Input: part model. Units: mm. Frame: model coordinates. A direction names the side the tool comes from. Give positions to 0.01 mm unless a question says otherwise; leave off trailing zeros. Loops run counter-clockwise (first coordinate to the right, second up) from the corner with the lowest first, then second, coordinate; pieces in that order, holes last.
Solid Edge part; units mm, degrees
sketch "Sketch1" plane through (0, 0, 25) normal (0, 0, 1) x (1, 0, 0)
  line L0 (-49.5, -36.5) -> (-19.5, -36.5)
  line L1 (-19.5, 6.5) -> (-19.5, -36.5)
  line L2 (-19.5, 6.5) -> (-49.5, 6.5)
  line L3 (-49.5, 6.5) -> (-49.5, -36.5)
  circle A0 centre (-25, -31) radius 2.2
  circle A1 centre (-44, 1) radius 2.2
  circle A2 centre (-25, 1) radius 2.2
  circle A3 centre (-44, -31) radius 2.2
extrude "ExtrudedProtrusion_1" add sketch "Sketch1" along normal blind 15
sketch "Sketch2" plane through (-34.5, -36.5, 32.5) normal (0, -1, 0) x (0, 0, 1)
  circle A0 centre (-7.5, 0) radius 4
extrude "Cutout1" cut sketch "Sketch2" against normal through all
sketch "Sketch3" plane through (-34.5, -36.5, 32.5) normal (0, -1, 0) x (1, 0, 0)
  line L0 (-5, 7.5) -> (-5, 4.5)
  line L1 (-5, 4.5) -> (5, 4.5)
  line L2 (5, 7.5) -> (5, 4.5)
  dimension "D1" = 5
  dimension "D2" = 5
extrude "Cutout2" cut sketch "Sketch3" against normal through all material side at (-39.45, -36.5, 38.5)
sketch "Sketch4" plane through (-24.5, -15, 40) normal (0, 0, 1) x (0, 1, 0)
  line L0 (-10.5, 25) -> (-10.5, 12.5)
extrude "Cutout3" cut sketch "Sketch4" against normal through all material side at (-43.25, -25.45, 40)
fillet "Round_1" radius 1 2 edges at (-39.5, -31, 37) (-29.5, -31, 37)
sketch "Sketch5" plane through (-44.5, -31, 40) normal (0, 0, 1) x (1, 0, 0)
  line L0 (0.5, 0) -> (2.0825, 1.5282)
  line L1 (2.0825, 1.5282) -> (0.5, 3.167)
  line L2 (0.5, 3.167) -> (-1.0825, 1.5282)
  line L3 (-1.0825, 1.5282) -> (0.5, 0)
  line L4 (19.5, 0) -> (21.0825, 1.5282)
  line L5 (21.0825, 1.5282) -> (19.5, 3.167)
  line L6 (19.5, 3.167) -> (17.9175, 1.5282)
  line L7 (17.9175, 1.5282) -> (19.5, 0)
extrude "Cutout4" cut sketch "Sketch5" against normal through all
properties material "ABS Plastic, medium impact"
(1) Cut plane A-A (z = 32). Return the cut outline in (x, y), and give its area (3 significant figures).
Values follow:
outline: (-49.5, -36.5) - (-19.5, -36.5) - (-19.5, -25.5) - (-49.5, -25.5) - close; hole (-45.57, -29.46) arc R2.2 ccw (long way) to (-42.43, -29.46) - (-44, -27.83) - close; hole (-26.57, -29.46) arc R2.2 ccw (long way) to (-23.43, -29.46) - (-25, -27.83) - close
area: 297 mm2
(2) Pin query (flat end, axial travel): pin 1 Ø2 at (x, y) = (-32.5, -29) entering from -Z; pin 2 Ø1.5 at (x, y) = (-35, -35) entering from +Z. Return the tip coordinate at first contact, or that it passes through.
Values follow:
pin 1: stops at z = 27.65
pin 2: stops at z = 37
(3) Cut plane B-B (y = -31). Return the cut outline in (x, z), and give its area (3 significant figures).
Values follow:
outline: (-49.5, 25) - (-46.2, 25) - (-46.2, 40) - (-49.5, 40) - close; (-41.8, 25) - (-38.5, 25) arc R4 cw to (-30.5, 25) - (-27.2, 25) - (-27.2, 40) - (-29.5, 40) - (-29.5, 38) arc R1 cw to (-30.5, 37) - (-38.5, 37) arc R1 cw to (-39.5, 38) - (-39.5, 40) - (-41.8, 40) - close; (-22.8, 25) - (-19.5, 25) - (-19.5, 40) - (-22.8, 40) - close
area: 263 mm2
(4) Ray query, probe 1 along X at (y, z) = (-31, 31.5); probe 2 along X at (y, z) = (-29.75, 26); probe 3 along X at (y, z) = (-31, 37.75). Return the intervals inside material, ascending.
Values follow:
probe 1: x = -49.5 to -46.2, -41.8 to -27.2, -22.8 to -19.5
probe 2: x = -49.5 to -45.81, -42.19 to -38.37, -30.63 to -26.81, -23.19 to -19.5
probe 3: x = -49.5 to -46.2, -41.8 to -39.47, -29.53 to -27.2, -22.8 to -19.5
(5) Cut plane C-C (z = 27.5). Return the cut outline in (x, y).
Values follow:
outline: (-49.5, -36.5) - (-37.62, -36.5) - (-37.62, -25.5) - (-49.5, -25.5) - close; (-31.38, -36.5) - (-19.5, -36.5) - (-19.5, -25.5) - (-31.38, -25.5) - close; hole (-45.57, -29.46) arc R2.2 ccw (long way) to (-42.43, -29.46) - (-44, -27.83) - close; hole (-26.57, -29.46) arc R2.2 ccw (long way) to (-23.43, -29.46) - (-25, -27.83) - close
(6) Cut plane D-D (y = -27.5). Return the cut outline in (x, z).
Values follow:
outline: (-49.5, 25) - (-38.5, 25) arc R4 cw to (-30.5, 25) - (-19.5, 25) - (-19.5, 40) - (-29.5, 40) - (-29.5, 38) arc R1 cw to (-30.5, 37) - (-38.5, 37) arc R1 cw to (-39.5, 38) - (-39.5, 40) - (-49.5, 40) - close
(7) Reachability of faces 1 (the flat face through (-29.5, -31, 39)), 2 (the flat face through (-25.77, -28.63, 32.61)), 3 (the flat face through (-19.5, -31, 32)) from +Z, -Z, +X, -X, +Y, -Y: full face, straight path, thin tool, end or side. Return the list, or none.
Values follow:
face 1: +Z, +Y, -Y
face 2: +Z, -Z
face 3: +Z, -Z, +X, +Y, -Y
